Input: part model. Units: mm. Frame: model coordinates. A direction names the side the tool comes from. Coordinates: 2 decimals unless noted, no trailing zeros. Loops run counter-clockwise (first coordinate to the right, second up) from the corner with the lowest first, then second, coordinate; pieces in that order, holes last.
```python
from build123d import *

# Parameters (mm, degrees)
PAD001005_DEPTH = 6.5
PAD001007_DEPTH = 8
SKETCH034_W     = 16
SKETCH034_H     = 2.5
POCKET024_DEPTH = 12.501
SKETCH036_W     = 10
SKETCH036_H     = 10
POCKET025_DEPTH = 12.501
SKETCH035_W     = 13
SKETCH035_H     = 13
POCKET026_DEPTH = 12.501
SKETCH033_R     = 2.25
PAD001006_DEPTH = 1.5
SKETCH032_R     = 2.25
PAD001004_DEPTH = 1.5
SKETCH006_R     = 2.325
POCKET023_DEPTH = 16.001
SKETCH030_W     = 10.3
SKETCH030_H     = 10
POCKET022_DEPTH = 16.276


with BuildPart() as inner_room_male:
    # Sketch029 → Pad001005 (new body, symmetric)
    with BuildSketch(Plane.XZ):
        with BuildLine():
            ThreePointArc((13, 6.45), (6.55, 0), (13, -6.45))
            Line((13, 6.45), (13, -6.45))
        make_face()
    extrude(amount=PAD001005_DEPTH, both=True)


with BuildPart() as cable_chain_link:
    # Sketch031 → Pad001007 (new body, symmetric)
    with BuildSketch(Plane.XZ):
        with BuildLine():
            ThreePointArc((0.325, 6.25), (-5.925, 0), (0.325, -6.25))
            Line((0.325, -6.25), (12.675, -6.25))
            ThreePointArc((12.675, -6.25), (18.925, 0), (12.675, 6.25))
            Line((0.325, 6.25), (12.675, 6.25))
        make_face()
    extrude(amount=PAD001007_DEPTH, both=True)

    # Sketch034 (on Face4 of Pad001007) → Pocket024 (cut, through all)
    with BuildSketch(Plane(origin=(0, 0, 6.25), x_dir=(-1, 0, 0), z_dir=(0, 0, 1))):
        Polygon((9.55, 8), (9.55, 6.5), (-6.45, 6.5), (-6.45, 8), (-6.45, 9), (9.55, 9), align=None)
        with Locations((1.55, -7.75)):
            Rectangle(SKETCH034_W, SKETCH034_H)
    extrude(amount=-POCKET024_DEPTH, mode=Mode.SUBTRACT)

    # Sketch036 (on Face5 of Pocket024) → Pocket025 (cut, through all)
    with BuildSketch(Plane(origin=(0, 0, 6.25), x_dir=(-1, 0, 0), z_dir=(0, 0, 1))):
        with Locations((2.15, 0)):
            Rectangle(SKETCH036_W, SKETCH036_H)
    extrude(amount=-POCKET025_DEPTH, mode=Mode.SUBTRACT)

    # Sketch035 (on Face4 of Pocket025) → Pocket026 (cut, through all)
    with BuildSketch(Plane(origin=(0, 0, 6.25), x_dir=(-1, 0, 0), z_dir=(0, 0, 1))):
        with Locations((-16.85, 0)):
            Rectangle(SKETCH035_W, SKETCH035_H)
    extrude(amount=-POCKET026_DEPTH, mode=Mode.SUBTRACT)

    # Sketch033 (on Face14 of Pocket026) → Pad001006 (new body)
    with BuildSketch(Plane.XZ.offset(6.5)):
        Circle(SKETCH033_R)
    extrude(amount=PAD001006_DEPTH)

    # Sketch032 (on Face5 of Pad001006) → Pad001004 (new body)
    with BuildSketch(Plane(origin=(0, 6.5, 0), x_dir=(1, 0, 0), z_dir=(0, 1, 0))):
        Circle(SKETCH032_R)
    extrude(amount=PAD001004_DEPTH)

    # Sketch006 (on Face6 of Pad001004) → Pocket023 (cut, through all)
    with BuildSketch(Plane(origin=(0, 8, 0), x_dir=(1, 0, 0), z_dir=(0, 1, 0))):
        with Locations((13, 0)):
            Circle(SKETCH006_R)
    extrude(amount=-POCKET023_DEPTH, mode=Mode.SUBTRACT)

    # Sketch030 (on Face9 of Pocket023) → Pocket022 (cut, through all)
    with BuildSketch(Plane(origin=(10.35, 0, 0), x_dir=(0, 0, 1), z_dir=(1, 0, 0))):
        Rectangle(SKETCH030_W, SKETCH030_H)
    extrude(amount=-POCKET022_DEPTH, mode=Mode.SUBTRACT)

    # Cut003003: cut inner-room-male
    add(inner_room_male.part, mode=Mode.SUBTRACT)


solid = cable_chain_link.part
```
Item 1: Contact query for flat-ended pins moving along their axis: P1, Ø6, axis at y = 5.5, z = -2, coming from the -X side (3 decimals); P2, Ø4, axis at x = 3, z = -3.5, coming from the +Y side; P3, Ø0.8, axis at y = 7.5, z = 3, coming from the -X side; P4, Ø1.2, axis at y = 1, z = 5.5, coming from the -X side. Output: stop coordinate, or through.
Result:
P1: stops at x = -5.925
P2: stops at y = 6.5
P3: stops at x = 6.45
P4: stops at x = 2.85
Item 2: Section query B-B (x = 3.75). Output: boundary loops of the cut face in (y, z).
Result:
outline: (-6.5, -6.25) - (6.5, -6.25) - (6.5, 6.25) - (-6.5, 6.25) - close; hole (-5, -5.15) - (5, -5.15) - (5, 5.15) - (-5, 5.15) - close
Item 3: Mould query, pull axis X, two halves, no side actions, for faces 1 (the face through (-0.29, -7.24, 2.23)), 2 (the face through (6, 0, -5.15)), 3 (the face through (-5.923, 5.74, 0.137)), 4 (the face through (18.923, 7.24, -0.137)). Classes: +X half, -X half, draft (parallel to the pull), parting line (faces both ways), or undercut.
Result:
face 1: undercut
face 2: draft
face 3: -X half
face 4: +X half
Item 4: Reachability of faces 5 (the face through (3, -6.5, 0)), 6 (the face through (6.45, -7, 0)), 7 (the face through (2.85, 0, -6)) from +Z, -Z, +X, -X, +Y, -Y: full face, straight path, thin tool, end or side. Return the list, or none.
Result:
face 5: -Y
face 6: +Z, -Z, -Y
face 7: +Z, -Z, -X
Item 5: Line query: L1, parallel to X at y = 7.1, z = 0 (3 decimals); L2, parallel to Y at x = 1, z = -1.5; L3, parallel to Y at x = 8.25, z = -0.25. Output: solid intervals per line, ascending.
Result:
L1: x = -2.25 to 2.25, 6.45 to 10.675, 15.325 to 18.925
L2: y = -8 to -5, 5 to 8
L3: y = -8 to -6.5, 6.5 to 8
Item 6: Section query D-D (x = -1.5). Output: boundary loops of the cut face in (y, z).
Result:
outline: (-8, -1.68) - (-6.5, -1.68) - (-6.5, -5.98) - (-5, -5.98) - (-5, 5.98) - (-6.5, 5.98) - (-6.5, 1.68) - (-8, 1.68) - close; (5, -5.98) - (6.5, -5.98) - (6.5, -1.68) - (8, -1.68) - (8, 1.68) - (6.5, 1.68) - (6.5, 5.98) - (5, 5.98) - close
Item 7: Section query A-A (z = 0). Count the separate pieces of the cut face and the enclosed holes in it, then the cut area to 3 significant figures.
Result:
separate pieces: 4
enclosed holes: 0
area: 74.4 mm2
Item 8: Section query C-C (y = -3.5). Output: boundary loops of the cut face in (x, z), then the cut area to 3 significant figures.
Result:
outline: (2.85, -6.25) - (10.35, -6.25) - (10.35, -5.88) arc R6.45 cw to (9.12, -5.15) - (2.85, -5.15) - close; (2.85, 5.15) - (9.12, 5.15) arc R6.45 cw to (10.35, 5.88) - (10.35, 6.25) - (2.85, 6.25) - close
area: 15.5 mm2
